Part model, mm, in its own coordinate system. Coordinates: 2 decimals unless noted, no trailing zeros. Order: outer loops, then holes, each group sorted by start corner. A loop starts at its lowest first (then second) coordinate and runs counter-clockwise, first axis right, second up.
from build123d import *

# Parameters (mm, degrees)
SKETCH_2_W         = 28.5
SKETCH_2_H         = 6
SKETCH_2_R         = 1.5
EXTRUDE_1_DEPTH    = 3
HOLE_WIZARD_M3_2_D = 2.5
CHAMFER_1_SIZE     = 0.5


with BuildPart() as part:
    # 草图2 → 凸台-拉伸1 (new body, symmetric)
    with BuildSketch(Plane.XY):
        with Locations((-11.25, 0)):
            Rectangle(SKETCH_2_W, SKETCH_2_H)
        with Locations((-15, 0)):
            Circle(SKETCH_2_R, mode=Mode.SUBTRACT)
        Circle(SKETCH_2_R, mode=Mode.SUBTRACT)
    extrude(amount=EXTRUDE_1_DEPTH, both=True)

    # M3 螺纹孔2 (through all)
    with Locations(Plane(origin=(0, 3, 0), x_dir=(1, 0, 0), z_dir=(0, 1, 0))):
        with Locations((-7.5, 0), (-22.5, 0)):
            Hole(HOLE_WIZARD_M3_2_D / 2)

    # 倒角1
    chamfer_1_edges = [part.edges().sort_by_distance(p)[0] for p in [
        (-11.25, -3, 3),
        (3, 0, 3),
        (-11.25, 3, 3),
        (3, 0, -3),
        (-11.25, -3, -3),
        (-25.5, 0, -3),
        (-11.25, 3, -3),
        (-25.5, 0, 3),
        (3, 3, 0),
        (3, -3, 0),
        (-25.5, -3, 0),
        (-25.5, 3, 0),
    ]]
    chamfer(chamfer_1_edges, length=CHAMFER_1_SIZE)


solid = part.part
Q1. Mould opens along Z. For faces 1 (the face through (-11, 0, 3)), 2 (the face through (-23.655, -0.042, 0.479)), 3 (the face through (-11, 3, 0)), 4 (the face through (-6.25, -0.04, -0.05)) say: pulls with the +Z half, pulls with the -Z half, needs draft (parallel to the pull), parting line crosses it, or undercut.
Results list:
face 1: pulls with the +Z half
face 2: undercut
face 3: needs draft
face 4: undercut
Q2. Cut at D-D on y = 2.25. Write the cut outline in (x, z).
Results list:
outline: (-25.5, -2.5) - (-25, -3) - (2.5, -3) - (3, -2.5) - (3, 2.5) - (2.5, 3) - (-25, 3) - (-25.5, 2.5) - close; hole circle Ø2.5 at (-22.5, 0); hole circle Ø2.5 at (-7.5, 0)
Q3. Cut at A-A on z = 1. Write the cut outline in (x, y).
Results list:
outline: (-25.5, -2.5) - (-25, -3) - (-23.25, -3) - (-23.25, 3) - (-25, 3) - (-25.5, 2.5) - close; (-21.75, -3) - (-8.25, -3) - (-8.25, 3) - (-21.75, 3) - close; (-6.75, -3) - (2.5, -3) - (3, -2.5) - (3, 2.5) - (2.5, 3) - (-6.75, 3) - close; hole circle Ø3 at (-15, 0); hole circle Ø3 at (0, 0)
Q4. Cut at B-B on x = -7.5. Write the cut outline in (y, z).
Results list:
outline: (-3, -2.5) - (-2.5, -3) - (2.5, -3) - (3, -2.5) - (3, -1.25) - (-3, -1.25) - close; (-3, 1.25) - (3, 1.25) - (3, 2.5) - (2.5, 3) - (-2.5, 3) - (-3, 2.5) - close
Q5. Wall check: line 1 along Z through (x, y) = (-22.5, -1); line 2 along Y through (x, z) = (-15, -1.1); line 3 along X through (y, z) = (-1, -1.5). Give the ranges that are in metal, low to high.
Results list:
line 1: z = -3 to -1.25, 1.25 to 3
line 2: y = -3 to -1.5, 1.5 to 3
line 3: x = -25.5 to -16.12, -13.88 to -1.12, 1.12 to 3
Q6. Pin check, flat tip, straight feed: pin 1 Ø3 at (x, z) = (-22.5, 0) entering from +Y. Stop position of the tip, or through.
Results list:
pin 1: stops at y = 3
Q7. Cut at C-C on y = 0. Write the cut outline in (x, z), and give its area (3 significant figures).
Results list:
outline: (-25.5, -2.5) - (-25, -3) - (-16.5, -3) - (-16.5, 3) - (-25, 3) - (-25.5, 2.5) - close; (-13.5, -3) - (-1.5, -3) - (-1.5, 3) - (-13.5, 3) - close; (1.5, -3) - (2.5, -3) - (3, -2.5) - (3, 2.5) - (2.5, 3) - (1.5, 3) - close; hole circle Ø2.5 at (-22.5, 0); hole circle Ø2.5 at (-7.5, 0)
area: 125 mm2
